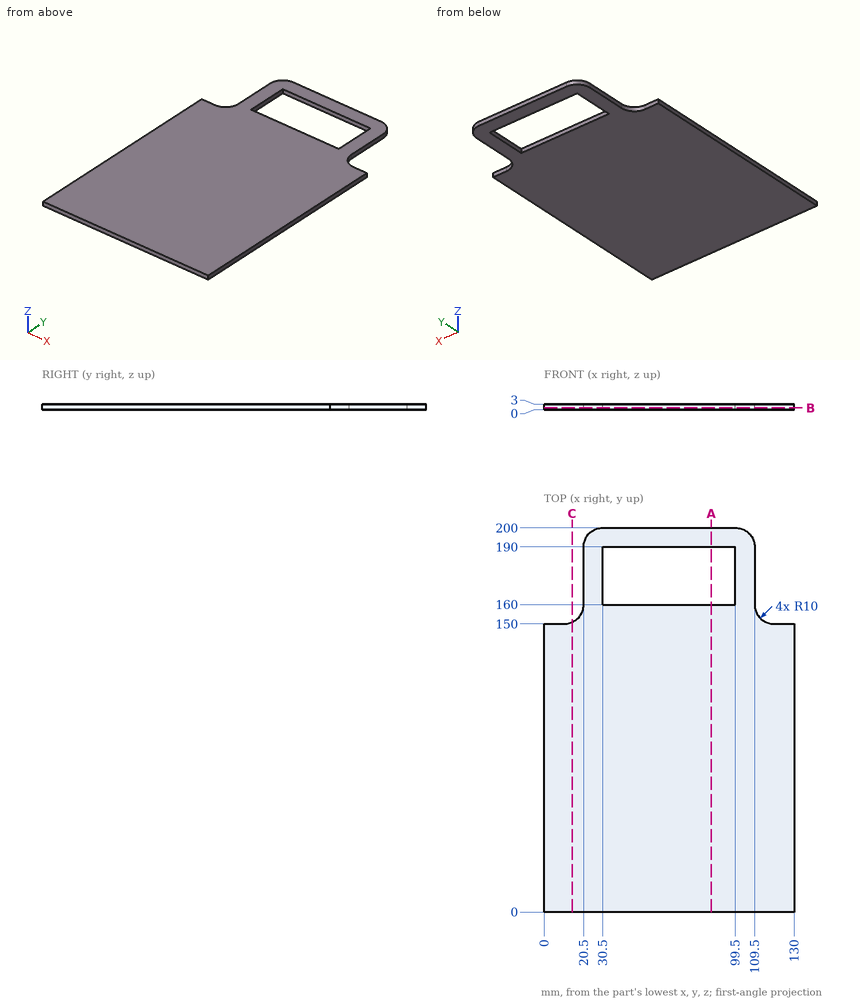
Here's the drawing with two shaded views (mm, measured from the low corner). I have some questions. Coordinates: 2 decimals unless noted, no trailing zeros. Order: outer loops, then holes, each group sorted by start corner. A loop starts at its lowest first (then second) coordinate and runs counter-clockwise, first axis right, second up.
Item 1: I'm going to push flat-ended pins straight in: pin 1 Ø0.9 at (y, z) = (173, 2) entering from -X; pin 2 Ø1.5 at (y, z) = (181.5, 1.5) entering from +X; pin 3 Ø0.9 at (x, z) = (124.5, 1.5) entering from +Y. Where does each tip first touch, or does it pass through?
Response values:
pin 1: stops at x = 20.5
pin 2: stops at x = 109.5
pin 3: stops at y = 150
Item 2: If we section it at A-A, the plane x = 87: List the corners of the cut face in (y, z) for me.
Response values:
outline: (0, 0) - (160, 0) - (160, 3) - (0, 3) - close; (190, 0) - (200, 0) - (200, 3) - (190, 3) - close
Item 3: I need wall thicknesses on probe 1 along Y at (x, z) = (64, 1.9); probe 2 along Y at (x, z) = (121, 2.1); probe 3 along Y at (x, z) = (27, 1.75). Which ranges of each line are inside material? Lowest first, please.
Response values:
probe 1: y = 0 to 160, 190 to 200
probe 2: y = 0 to 150
probe 3: y = 0 to 199.37
Item 4: If we section it at C-C, the plane x = 14.5: List the corners of the cut face in (y, z) for me, then the cut area to 3 significant figures.
Response values:
outline: (0, 0) - (150.83, 0) - (150.83, 3) - (0, 3) - close
area: 453 mm2
Item 5: If we section it at B-B, the plane z = 0.95: List the corners of the cut face in (x, y) for me, then the cut area to 3 significant figures.
Response values:
outline: (0, 0) - (130, 0) - (130, 150) - (119.5, 150) arc R10 cw to (109.5, 160) - (109.5, 190) arc R10 ccw to (99.5, 200) - (30.5, 200) arc R10 ccw to (20.5, 190) - (20.5, 160) arc R10 cw to (10.5, 150) - (0, 150) - close; hole (30.5, 160) - (99.5, 160) - (99.5, 190) - (30.5, 190) - close
area: 21,900 mm2
